Job drawing, mm, ordinate dimensions from the low corner. One solid piece. Give positions to 0.01 mm unless a question says otherwise; leave off trailing zeros. Order: outer loops, then holes, each group sorted by start corner. A loop starts at its lowest first (then second) coordinate and runs counter-clockwise, first axis right, second up.
Item 1: Flat gauge pins, fed straight in: P1, Ø3, axis at x = 2.5, z = 3, coming from the -Y side; P2, Ø5, axis at y = 25, z = 1.5, coming from the -X side; P3, Ø2, axis at y = 40.5, z = 1.5, coming from the -X side; P4, Ø5, axis at x = 18.5, z = 6, coming from the +Y side. Where does each tip first touch, or does it go through?
Item 2: Band-saw the part on B-B on z = 5. Give the cut face in (x, y).
Item 3: Band-saw the part on C-C on x = 38. Give the cut face in (y, z), plus the area to 3 significant figures.
Item 4: Band-saw the part on D-D on y = 7. Give the cut face in (x, z), plus the area to 3 significant figures.
Item 5: Wall check: L1, parallel to Z at x = 4, y = 28.55; L2, parallel to Y at x = 38, z = 6.25; L3, parallel to X at y = 34.4, z = 5. Give the ranges that are in metal, low to high.
Item 6: Two-plate mould, pull along Y, no slides. Class the marked faces 1, 2 and 3: released by +Y, released by -Y, zero draft, split by the parting line, or undercut.
Item 7: Band-saw the part on A-A on x = 4. Give the cut face in (y, z).
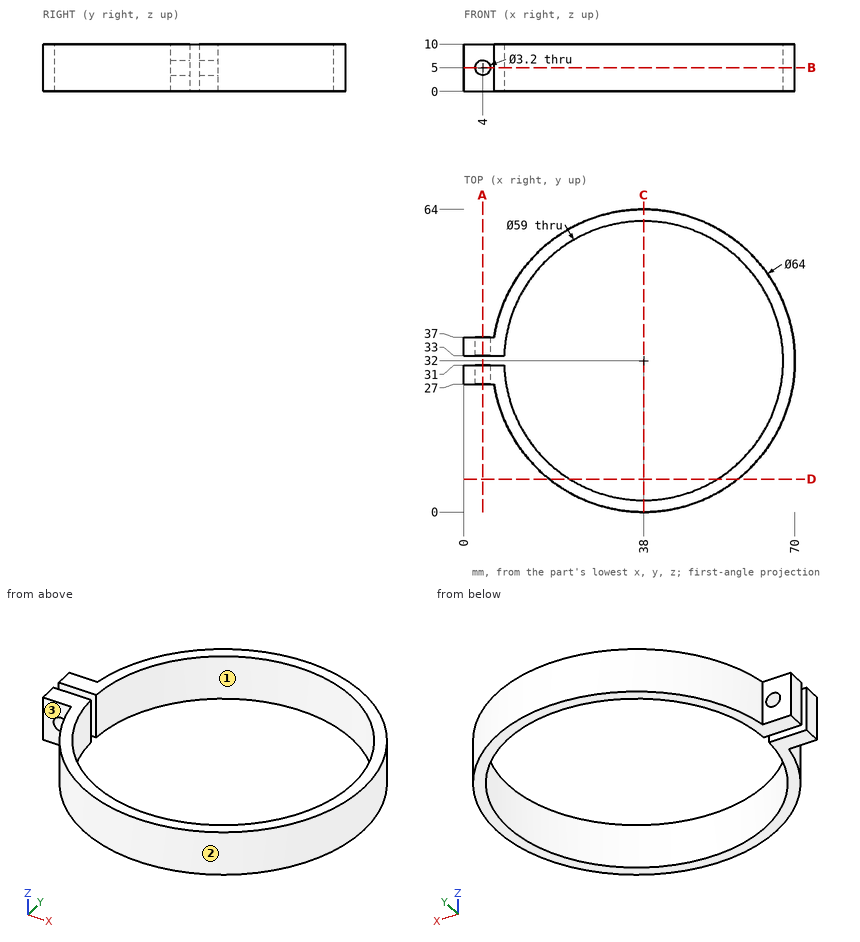
The answers:
1. P1: stops at y = 27
1. P2: stops at x = 0
1. P3: stops at x = 6.89
1. P4: stops at y = 59.11
2. outline: (0, 27) - (2.4, 27) - (2.4, 31) - (0, 31) - close; (0, 33) - (2.4, 33) - (2.4, 37) - (0, 37) - close; (5.6, 27) - (6.39, 27) arc R32 ccw (long way) to (6.39, 37) - (5.6, 37) - (5.6, 33) - (8.52, 33) arc R29.5 cw (long way) to (8.52, 31) - (5.6, 31) - close
3. outline: (0, 0) - (2.5, 0) - (2.5, 10) - (0, 10) - close; (61.5, 0) - (64, 0) - (64, 10) - (61.5, 10) - close
3. area: 50.0 mm2
4. outline: (18.03, 0) - (22.34, 0) - (22.34, 10) - (18.03, 10) - close; (53.66, 0) - (57.97, 0) - (57.97, 10) - (53.66, 10) - close
4. area: 86.3 mm2
5. L1: z = 0 to 3.4, 6.6 to 10
5. L2: y = 0 to 2.5, 61.5 to 64
5. L3: x = 0 to 2.4, 5.6 to 8.6, 67.4 to 69.91
6. face 1: undercut
6. face 2: split by the parting line
6. face 3: released by -Y
7. outline: (27, 0) - (31, 0) - (31, 3.4) - (27, 3.4) - close; (27, 6.6) - (31, 6.6) - (31, 10) - (27, 10) - close; (33, 0) - (37, 0) - (37, 3.4) - (33, 3.4) - close; (33, 6.6) - (37, 6.6) - (37, 10) - (33, 10) - close
